Source: CAD feature listing. Evaluate the final solid. Frame: model axes, mm. A direction names the side the tool comes from. Give positions to 0.01 mm unless a question says otherwise; leave off trailing zeros. Order: outer loops, then holes, each group sorted by start corner. A loop starts at its lowest first (then second) coordinate and runs counter-clockwise, first axis right, second up. Notation, with made-up numbers: M 27,-10 L 54,-10 A19 cw 54,3 Z; hole C 12,46 d11. An arc over 180 degrees is marked long. Use CSV: the item, a comma, the result in double quotes. Start each with the question number.
1. Line query: line 1 along X through (y, z) = (-3, -1); line 2 along Y through (x, z) = (8, -3.75); line 3 along Y through (x, z) = (-12.5, -5). Output: solid intervals per line, ascending. Write a range as [from, to].
2. Section query C-C, the plane y = -4. Return the cut outline in (x, z).
3. Section query B-B, the plane x = 0.8. Return the cut outline in (y, z), plus the area to 4 significant figures.
4. Section query A-A, the plane x = -13. Return the cut outline in (y, z), plus the area to 3 significant figures.
5. Section query D-D, the plane z = -4.25. Return the cut outline in (x, y), plus the area to 3 significant figures.
6. Mould query, pull axis Y, two halves, no side actions, for faces 5 (the flat face through (-13, -17, 0)), 6 (the cylindrical face through (13.03, -5.58, 0.04)), 7 (the flat face through (0, -23, 0)), 8 (the flat face through (-13, -6.8, 0)). Classes: released by +Y, released by -Y, zero draft, split by the parting line, or undercut.
7. Pin query (flat end, axial travel): P1, Ø2, axis at y = -2, z = 2.5, coming from the -X side; P2, Ø0.8, axis at x = -13, y = -17.5, coming from the +Z side; P3, Ø3.5, axis at x = 7, z = -0.5, coming from the +Y side. Return the tip coordinate at first contact, or that it passes through.
8. Reachability of faces 1 (the flat face through (-13, -17.5, 1.5)), 2 (the flat face through (16, -6, -0.5)), 3 (the flat face through (11.5, -15, 0)), 4 (the flat face through (-13, -17.5, -1.5)) from +Z, -Z, +X, -X, +Y, -Y: full face, straight path, thin tool, end or side. Return the list, or none.
from build123d import *

# Parameters (mm, degrees)
SKETCH2_W           = 23
SKETCH2_H           = 12
BOSS_EXTRUDE1_DEPTH = 23
BOSS_EXTRUDE2_START = -4.4
BOSS_EXTRUDE2_DEPTH = 2.4
SKETCH4_R           = 6
SKETCH4_R_2         = 2.5
BOSS_EXTRUDE3_DEPTH = 3.5
BOSS_EXTRUDE4_DEPTH = 3
SKETCH6_W           = 3
SKETCH6_H           = 1
BOSS_EXTRUDE5_DEPTH = 3
SKETCH7_R           = 2.5
BOSS_EXTRUDE6_DEPTH = 3


with BuildPart() as part:
    # Sketch2 → Boss-Extrude1 (new body)
    with BuildSketch(Plane(origin=(0, 0, 0), x_dir=(1, 0, 0), z_dir=(0, 1, 0))):
        Rectangle(SKETCH2_W, SKETCH2_H)
    extrude(amount=-BOSS_EXTRUDE1_DEPTH)

    # Sketch3 → Boss-Extrude2 (add)
    with BuildSketch(Plane(origin=(0, 0, 0), x_dir=(1, 0, 0), z_dir=(0, 1, 0)).offset(BOSS_EXTRUDE2_START)):
        with BuildLine():
            Line((-16.2, -0.5), (-16.2, -6))
            Line((-16.2, -6), (-11.5, -6))
            Line((-11.5, -6), (-11.5, 6))
            Line((-11.5, 6), (-16.2, 6))
            Line((-16.2, 6), (-16.2, 0.5))
            Line((-16.2, 0.5), (-15.584293743, 0.5))
            ThreePointArc((-15.584293743, 0.5), (-14.459449294, 0.965925826), (-13.718268339, 0))
            ThreePointArc((-13.718268339, 0), (-14.459449294, -0.965925826), (-15.584293743, -0.5))
            Line((-15.584293743, -0.5), (-16.2, -0.5))
        make_face()
        with BuildLine():
            Line((11.5, 6), (11.5, -6))
            Line((11.5, -6), (16.2, -6))
            Line((16.2, -6), (16.2, -0.5))
            Line((16.2, -0.5), (14.894380034, -0.5))
            ThreePointArc((14.894380034, -0.5), (13.02835463, 0), (14.894380034, 0.5))
            Line((14.894380034, 0.5), (16.2, 0.5))
            Line((16.2, 0.5), (16.2, 6))
            Line((16.2, 6), (11.5, 6))
        make_face()
    extrude(amount=-BOSS_EXTRUDE2_DEPTH)

    # Sketch4 → Boss-Extrude3 (add)
    with BuildSketch(Plane(origin=(0, 0, 0), x_dir=(1, 0, 0), z_dir=(0, 1, 0))):
        with Locations((-5.5, 0)):
            Circle(SKETCH4_R)
        with Locations((0.8, 0)):
            Circle(SKETCH4_R_2)
    extrude(amount=BOSS_EXTRUDE3_DEPTH)

    # Sketch5 → Boss-Extrude4 (add)
    with BuildSketch(Plane(origin=(0, 3.5, 0), x_dir=(1, 0, 0), z_dir=(0, 1, 0))):
        Polygon((-3.255005568, -0.15), (-3.437184296, 0), (-3.255005568, 0.15), (-3.455589794, 0.274946425), (-3.295142762, 0.44844683), (-3.51047784, 0.544986424), (-3.374587739, 0.738324266), (-3.600868956, 0.805301127), (-3.491960749, 1.015026288), (-3.725150111, 1.051245213), (-3.645167266, 1.273615142), (-3.881103504, 1.278429803), (-3.831473318, 1.509476304), (-4.065946143, 1.482800783), (-4.047554268, 1.718400825), (-4.276379508, 1.660711148), (-4.289554146, 1.896660443), (-4.508648409, 1.808986083), (-4.553154459, 2.04107411), (-4.758608002, 1.924979619), (-4.833651254, 2.149064761), (-5.021797754, 2.006621847), (-5.126039057, 2.218705301), (-5.293521035, 2.052455862), (-5.425100203, 2.248752992), (-5.568928939, 2.061663752), (-5.725497937, 2.238671633), (-5.843106805, 2.034081205), (-6.021871655, 2.188641125), (-6.111161921, 1.97020043), (-6.308932561, 2.099554265), (-6.368310838, 1.871161381), (-6.581558046, 1.973000809), (-6.609964728, 1.738731414), (-6.834883102, 1.811239107), (-6.831811271, 1.575273743), (-7.064387138, 1.6171558), (-7.02989161, 1.383705275), (-7.265974648, 1.39421431), (-7.200670997, 1.167444554), (-7.436048299, 1.146393032), (-7.34110187, 0.930350756), (-7.571573122, 0.878114343), (-7.448678237, 0.676654828), (-7.670130674, 0.594165683), (-7.521480394, 0.410883978), (-7.729962192, 0.299614123), (-7.558209186, 0.137780894), (-7.749999982, -0.000284059), (-7.558209186, -0.137780894), (-7.729886469, -0.300177172), (-7.521480394, -0.410883978), (-7.669980579, -0.594713616), (-7.448678237, -0.676654828), (-7.571351335, -0.878637381), (-7.34110187, -0.930350756), (-7.435758777, -1.146881842), (-7.200670997, -1.167444554), (-7.265622557, -1.394660168), (-7.02989161, -1.383705275), (-7.063978761, -1.617550752), (-6.831811271, -1.575273743), (-6.834425728, -1.811576103), (-6.609964728, -1.738731414), (-6.581059835, -1.973273836), (-6.368310838, -1.871161381), (-6.308402404, -2.099758451), (-6.111161921, -1.97020043), (-6.021319013, -2.188772827), (-5.843106805, -2.034081205), (-5.724932672, -2.238728499), (-5.568928939, -2.061663752), (-5.424532402, -2.248734009), (-5.293521035, -2.052455862), (-5.125478853, -2.218610806), (-5.021797754, -2.006621847), (-4.833108643, -2.148896442), (-4.758608002, -1.924979619), (-4.552639125, -2.040834969), (-4.508648409, -1.808986083), (-4.289075284, -1.896354748), (-4.276379508, -1.660711148), (-4.047120423, -1.718034032), (-4.065946143, -1.482800783), (-3.831092233, -1.509054958), (-3.881103504, -1.278429803), (-3.644845742, -1.273146762), (-3.725150111, -1.051245213), (-3.491704522, -1.014519232), (-3.600868956, -0.805301127), (-3.374401382, -0.737787582), (-3.51047784, -0.544986424), (-3.295029601, -0.447890096), (-3.455589794, -0.274946425), align=None)
    extrude(amount=BOSS_EXTRUDE4_DEPTH)

    # Sketch6 → Boss-Extrude5 (add)
    with BuildSketch(Plane.ZY.offset(11.5)):
        with Locations((0, -17.5)):
            Rectangle(SKETCH6_W, SKETCH6_H)
    extrude(amount=BOSS_EXTRUDE5_DEPTH)

    # Sketch7 → Boss-Extrude6 (add, symmetric)
    with BuildSketch(Plane(origin=(0, 6.5, 0), x_dir=(1, 0, 0), z_dir=(0, 1, 0))):
        with Locations((-5.5, 0)):
            Circle(SKETCH7_R)
    extrude(amount=BOSS_EXTRUDE6_DEPTH, both=True)


solid = part.part
Result set:
1,line 1,"[-11.5, 11.5]"
1,line 2,"[-23, 0]"
1,line 3,"[-6.8, -4.4]"
2,outline,"M -11.5,-6 L 11.5,-6 L 11.5,6 L -11.5,6 Z"
3,outline,"M -23,-6 L 0,-6 L 0,-2.5 L 3.5,-2.5 L 3.5,2.5 L 0,2.5 L 0,6 L -23,6 Z"
3,area,"293.5 mm2"
4,outline,"M -18,-1.5 L -17,-1.5 L -17,1.5 L -18,1.5 Z; M -6.8,-6 L -4.4,-6 L -4.4,6 L -6.8,6 Z"
4,area,"31.8 mm2"
5,outline,"M -16.2,-6.8 L -11.5,-6.8 L -11.5,-23 L 11.5,-23 L 11.5,-6.8 L 16.2,-6.8 L 16.2,-4.4 L 11.5,-4.4 L 11.5,0 L -1.26,0 L -1.26,3.5 L -9.74,3.5 L -9.74,0 L -11.5,0 L -11.5,-4.4 L -16.2,-4.4 Z"
5,area,"581 mm2"
6,face 5,"undercut"
6,face 6,"zero draft"
6,face 7,"released by -Y"
6,face 8,"undercut"
7,P1,"x = -11.5"
7,P2,"z = 1.5"
7,P3,"y = 0"
8,face 1,"+Z, -X, -Y"
8,face 2,"+X, +Y, -Y"
8,face 3,"+Z, -Z, +X, -Y"
8,face 4,"-Z, -X, -Y"
